CAD build for the part. Positions are in the model's coordinates, mm. Give positions to 0.01 mm unless a question says otherwise; leave off trailing zeros. Order: outer loops, then holes, each group sorted by start corner. A loop starts at its lowest first (then second) coordinate and runs counter-clockwise, first axis right, second up.
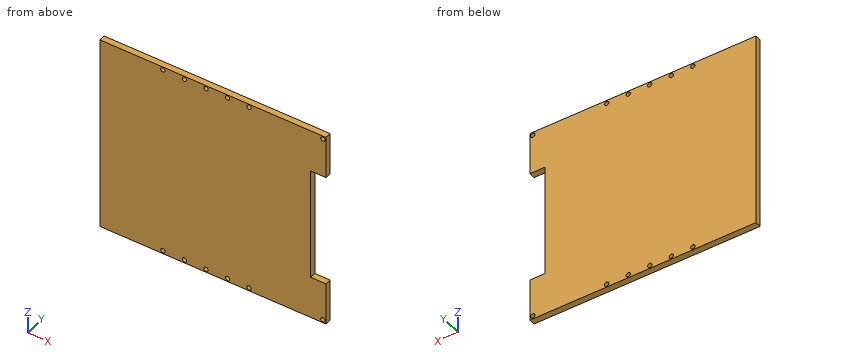
```python
from build123d import *

# Parameters (mm, degrees)
SKETCH1_W           = 183.77
SKETCH1_H           = 158
SKETCH1_R           = 1.75
BOSS_EXTRUDE1_DEPTH = 5
SKETCH2_W           = 25
SKETCH2_H           = 90
CUT_EXTRUDE1_DEPTH  = 10


with BuildPart() as part:
    # Sketch1 → Boss-Extrude1 (new body)
    with BuildSketch(Plane(origin=(0, 0, 0), x_dir=(1, 0, 0), z_dir=(0, 1, 0))):
        Rectangle(SKETCH1_W, SKETCH1_H)
        with Locations(Location((89.385, 76.5, 0), (0, 0, 270))):
            Circle(SKETCH1_R, mode=Mode.SUBTRACT)
        with Locations(Location((29.385, 76.5, 0), (0, 0, 270))):
            Circle(SKETCH1_R, mode=Mode.SUBTRACT)
        with Locations(Location((11.885, 76.5, 0), (0, 0, 270))):
            Circle(SKETCH1_R, mode=Mode.SUBTRACT)
        with Locations(Location((-5.615, 76.5, 0), (0, 0, 270))):
            Circle(SKETCH1_R, mode=Mode.SUBTRACT)
        with Locations(Location((-23.115, 76.5, 0), (0, 0, 270))):
            Circle(SKETCH1_R, mode=Mode.SUBTRACT)
        with Locations(Location((-40.615, 76.5, 0), (0, 0, 270))):
            Circle(SKETCH1_R, mode=Mode.SUBTRACT)
        with Locations(Location((89.385, -76.5, 0), (0, 0, 270))):
            Circle(SKETCH1_R, mode=Mode.SUBTRACT)
        with Locations(Location((29.385, -76.5, 0), (0, 0, 270))):
            Circle(SKETCH1_R, mode=Mode.SUBTRACT)
        with Locations(Location((11.885, -76.5, 0), (0, 0, 270))):
            Circle(SKETCH1_R, mode=Mode.SUBTRACT)
        with Locations(Location((-5.615, -76.5, 0), (0, 0, 270))):
            Circle(SKETCH1_R, mode=Mode.SUBTRACT)
        with Locations(Location((-23.115, -76.5, 0), (0, 0, 270))):
            Circle(SKETCH1_R, mode=Mode.SUBTRACT)
        with Locations(Location((-40.615, -76.5, 0), (0, 0, 270))):
            Circle(SKETCH1_R, mode=Mode.SUBTRACT)
    extrude(amount=BOSS_EXTRUDE1_DEPTH)

    # Sketch2 → Cut-Extrude1 (cut)
    with BuildSketch(Plane(origin=(0, 5, 0), x_dir=(1, 0, 0), z_dir=(0, 1, 0))):
        with Locations((91.885, 0)):
            Rectangle(SKETCH2_W, SKETCH2_H)
    extrude(amount=-CUT_EXTRUDE1_DEPTH, mode=Mode.SUBTRACT)


solid = part.part
```
Item 1: Wall check: L1, parallel to Z at x = -23, y = 0.85; L2, parallel to X at y = 4.7, z = -28 (3 decimals); L3, parallel to Z at x = 81.5, y = 3.05. Give the ranges that are in metal, low to high.
Item 2: Slice it at A-A (y = 4.1). State how many separate pieces and enclosed holes the cut face has, and give its area (3 significant figures).
Item 3: Drop a flat-ended pin along its axis: pin 1 Ø2.5 at (y, z) = (3, -22.5) entering from +X (3 decimals). Give the stop position or say it passes through.
Item 4: Slice it at B-B (z = -4). Give the cut face in (x, y) (3 decimals), and give its area (3 significant figures).
A:
1. L1: z = -79 to -78.25, -74.75 to 74.75, 78.25 to 79
1. L2: x = -91.885 to 79.385
1. L3: z = -79 to -45, 45 to 79
2. separate pieces: 1
2. enclosed holes: 12
2. area: 27,800 mm2
3. pin 1: stops at x = 79.385
4. outline: (-91.885, 0) - (79.385, 0) - (79.385, 5) - (-91.885, 5) - close
4. area: 856 mm2
